Work out the finished part from the listing and answer in its coordinate system (mm). A direction names the side the tool comes from. Give positions to 0.01 mm unless a question says otherwise; leave off trailing zeros. Order: outer loops, then holes, each group sorted by start corner. A loop starts at its lowest first (then second) coordinate and runs counter-clockwise, first axis right, second up.
```python
from build123d import *

# Parameters (mm, degrees)
RECPAT_COUNT = 2
RECPAT_ANGLE = 90


with BuildPart() as part:
    # Fillet1: read off the stored shape, not the designer's step
    # Fillet1 outline → Fillet1 (revolve)
    with BuildSketch(Plane.YX):
        with BuildLine():
            Line((2, 3.25), (2, 8.05))
            Line((2, 8.05), (0, 8.05))
            Line((0, 8.05), (0, 2.05))
            Line((0, 2.05), (5, 2.05))
            Line((5, 2.05), (5, 3.05))
            Line((5, 3.05), (2.2, 3.05))
            ThreePointArc((2.2, 3.05), (2.058578644, 3.108578644), (2, 3.25))
        make_face()
    revolve(axis=Axis((0, 0, 0), (1, 0, 0)))

    # PanSke → Pan (revolve)
    with BuildSketch(Plane.XY, mode=Mode.PRIVATE) as pan_sk:
        with BuildLine():
            Line((2.05, 4.424646879), (2.05, 0))
            Line((2.05, 0), (0, 0))
            ThreePointArc((0, 0), (0.537396082, 2.438237068), (2.05, 4.424646879))
        make_face()
    revolve(pan_sk.sketch.rotate(Axis((0, 0, 0), (1, 0, 0)), 90), axis=Axis((0, 0, 0), (1, 0, 0)))

    # Sketch3 → Recess section 0
    with BuildSketch(Plane(origin=(0, 0, 0), x_dir=(0, 0, -1), z_dir=(1, 0, 0))):
        with BuildLine():
            Line((-0.515, 2.15), (0.515, 2.15))
            Line((0.515, 2.15), (0.515, -2.15))
            Line((0.515, -2.15), (-0.515, -2.15))
            Line((-0.515, -2.15), (-0.515, 2.15))
        make_face()
    # Sketch4 → Recess section 1
    with BuildSketch(Plane(origin=(2.34, 0, 0), x_dir=(0, 0, -1), z_dir=(1, 0, 0))):
        with BuildLine():
            Line((-0.515, 2.106524682), (0.515, 2.106524682))
            Line((0.515, 2.106524682), (0.515, -2.106524682))
            Line((0.515, -2.106524682), (-0.515, -2.106524682))
            Line((-0.515, -2.106524682), (-0.515, 2.106524682))
        make_face()
    recess = loft(mode=Mode.SUBTRACT)

    # RecPat: Recess ×2 about axis
    recpat_axis = Axis((0, 0, 0), (1, 0, 0))
    for i in range(1, RECPAT_COUNT):
        add(recess.rotate(recpat_axis, i * RECPAT_ANGLE / (RECPAT_COUNT - 1)), mode=Mode.SUBTRACT)

    # RecCorSke → RecessCore (revolve, cut)
    with BuildSketch(Plane.XY, mode=Mode.PRIVATE) as recesscore_sk:
        Polygon((0, 0), (0, 1.172663335), (4.6, 0.851), (4.876506661, 0), align=None)
    revolve(recesscore_sk.sketch.rotate(Axis((-3.175, 0, 0), (1, 0, 0)), 90), axis=Axis((-3.175, 0, 0), (1, 0, 0)), mode=Mode.SUBTRACT)


solid = part.part
```
1. The part is cut by section A-A (y = -4). Write down the section's boundary in (x, z), then the cut area to 3 significant figures.
Findings below:
outline: (2.05, -3) - (3.05, -3) - (3.05, 3) - (2.05, 3) - (2.05, 1.89) arc R4.2 ccw to (2.05, -1.89) - close
area: 7.15 mm2
2. The part is cut by section B-B (x = 7.5). Write down the section's boundary in (y, z), then the cut area to 3 significant figures.
Findings below:
outline: circle Ø4 at (0, 0)
area: 12.6 mm2
3. The part is cut by section D-D (y = 2.75). Write down the section's boundary in (x, z), then the cut area to 3 significant figures.
Findings below:
outline: (2.05, -4.18) - (3.05, -4.18) - (3.05, 4.18) - (2.05, 4.18) - (2.05, 3.47) arc R5.11 ccw to (2.05, -3.47) - close
area: 14.8 mm2
4. The mould has two halves that part along Z. Classify faces 1 (the face through (3.05, 2.2, -1)), 2 (the face through (4.863, -0.012, 0.039)), 3 (the face through (2.888, -0.656, -0.715)), 4 (the face through (2.56, -1.08, -4.88)): pulls with the +Z half, pulls with the -Z half, needs draft (parallel to the pull), parting line crosses it, or undercut.
Findings below:
face 1: needs draft
face 2: undercut
face 3: undercut
face 4: parting line crosses it
5. Straight lines are drawn through the part: probe 1 along Z at (x, y) = (7.75, 0); probe 2 along Y at (x, z) = (2.25, -1.25) (3 decimals); probe 3 along Z at (x, y) = (2, -1.25) (3 decimals). For each, find the intervals that lie inside material, in ascending order.
Findings below:
probe 1: z = -2 to 2
probe 2: y = -4.841 to -0.515, 0.515 to 4.841
probe 3: z = -4.2 to -0.515, 0.515 to 4.2
6. Which of the six approach directions +Z, -Z, +X, -X, +Y, -Y give full straight-line access (tool end or side, diameter ignored) to faces 5 (the face through (2.34, -1.5, 0)), 6 (the face through (8.05, 0, 0)), 7 (the face through (6, 0, -2))?
Findings below:
face 5: -X
face 6: +Z, -Z, +X, +Y, -Y
face 7: +X
7. The part is cut by section C-C (x = 2.5). Write down the section's boundary in (y, z), then the cut area to 3 significant figures.
Findings below:
outline: circle Ø10 at (0, 0); hole circle Ø2 at (0, 0)
area: 75.4 mm2
8. Given P1, Ø3, axis at x = 7, z = 1.5, coming from the +Y side; P2, Ø0.8, axis at y = 0, z = -1.5, coming from the -X side; P3, Ø1, axis at y = 2.5, z = 3, coming from the -X side, each flat-ended and moving along its own axis, determine where each tip first touches the part or whether it passes through.
Findings below:
P1: stops at y = 2
P2: stops at x = 2.34
P3: stops at x = 1.1
